Read the model definition and answer for the solid it produces. Units are mm, in the model's axes. Face numbers are marked on the shaded views. A direction names the side the tool comes from. Give positions to 0.01 mm unless a question says otherwise; leave off trailing zeros. Order: outer loops, then holes, each group sorted by start corner. A loop starts at its lowest first (then second) coordinate and runs counter-clockwise, first axis right, second up. Notation, with made-up numbers: (26, -2.75) - (35, -2.75) arc R12 ccw to (35, 9.25) - close; hole circle Ø9 at (83, -22.75). An arc over 180 degrees is marked (long way). Write each question's results on one line, items separated by ' | '. Start each with the question number.
Q1. Find section A-A on z = -10.5. Give the vertices of the cut face in (x, y), and give its area (3 significant figures).
Q2. Find section B-B on y = 61. Give the vertices of the cut face in (x, z).
Q3. Find section C-C on x = 5. Give the vertices of the cut face in (y, z).
Q4. Find the intervals of material crossed by line 1 along Z through (x, y) = (4.5, 40); line 2 along Y through (x, z) = (-10, 13.5); line 3 along Y through (x, z) = (18, 23), in increasing order. Write a range as from..to.
Q5. For a pull along Z with two mould halves and no side action, classify the marked faces 4, 5, 6 and 7 as +Z half, -Z half, draft (parallel to the pull), parting line (faces both ways), or undercut.
Q6. Flat-ended cylindrical pins translate along their axes: P1, Ø1, axis at x = -0.5, z = 36.5, coming from the -Y side; P2, Ø10, axis at x = -8, z = 63, coming from the +Y side; P3, Ø1, axis at x = -18, y = 23.5, coming from the -Z side. Find the tip coordinate at first contact, or state that the pin passes through.
Q7. Find section D-D on y = 40. Give the vertices of the cut face in (x, z), and give its area (3 significant figures).
Q8. A tool of negligible diameter and unlimited length cuts with its end or side. For the marked faces 1, 2 and 3, from which of +Z, -Z, +X, -X, +Y, -Y can it reach the whole face along a straight path? Write none if from no direction.
from build123d import *

# Parameters (mm, degrees)
SKETCH1_W           = 50
SKETCH1_H           = 50
BOSS_EXTRUDE1_DEPTH = 100
SKETCH2_W           = 50
SKETCH2_H           = 50
BOSS_EXTRUDE2_DEPTH = 50
CUT_EXTRUDE1_DEPTH  = 50
CUT_EXTRUDE3_DEPTH  = 25
CUT_EXTRUDE4_DEPTH  = 25
CUT_EXTRUDE5_REACH  = 52
SKETCH6_W           = 30
SKETCH6_H           = 30


with BuildPart() as part:
    # Sketch1 → Boss-Extrude1 (new body)
    with BuildSketch(Plane(origin=(0, 0, 0), x_dir=(1, 0, 0), z_dir=(0, 1, 0))):
        Rectangle(SKETCH1_W, SKETCH1_H)
    extrude(amount=BOSS_EXTRUDE1_DEPTH)

    # Sketch2 → Boss-Extrude2 (add)
    with BuildSketch(Plane.XY.offset(25)):
        with Locations((0, 50)):
            Rectangle(SKETCH2_W, SKETCH2_H)
    extrude(amount=BOSS_EXTRUDE2_DEPTH)

    # Sketch3 → Cut-Extrude1 (cut)
    with BuildSketch(Plane.XY.offset(75)):
        with BuildLine():
            Line((8.4e-08, 75), (-25, 75))
            Line((-25, 75), (-25, 49.999999966))
            ThreePointArc((-25, 49.999999966), (-17.677669512, 67.677669547), (8.4e-08, 75))
        make_face()
        with BuildLine():
            Line((25, 75), (8.4e-08, 75))
            ThreePointArc((8.4e-08, 75), (17.677669559, 67.6776695), (25, 50))
            Line((25, 50), (25, 75))
        make_face()
        with BuildLine():
            Line((25, 25), (25, 50))
            ThreePointArc((25, 50), (17.677669509, 32.32233045), (-5.8e-08, 25))
            Line((-5.8e-08, 25), (25, 25))
        make_face()
        with BuildLine():
            ThreePointArc((-5.8e-08, 25), (-17.677669538, 32.322330479), (-25, 49.999999966))
            Line((-25, 49.999999966), (-25, 25))
            Line((-25, 25), (-5.8e-08, 25))
        make_face()
    extrude(amount=-CUT_EXTRUDE1_DEPTH, mode=Mode.SUBTRACT)

    # Sketch4 → Cut-Extrude3 (cut)
    with BuildSketch(Plane(origin=(0, 100, 0), x_dir=(1, 0, 0), z_dir=(0, 1, 0))):
        with BuildLine():
            ThreePointArc((0, -25), (-17.67766954, -17.677669519), (-25, 3e-08))
            Line((-25, 3e-08), (-25, -25))
            Line((-25, -25), (0, -25))
        make_face()
        with BuildLine():
            Line((0, 25), (-25, 25))
            Line((-25, 25), (-25, 3e-08))
            ThreePointArc((-25, 3e-08), (-17.677669519, 17.67766954), (0, 25))
        make_face()
        with BuildLine():
            Line((25, 25), (0, 25))
            ThreePointArc((0, 25), (17.67766953, 17.67766953), (25, 0))
            Line((25, 0), (25, 25))
        make_face()
        with BuildLine():
            Line((25, -25), (25, 0))
            ThreePointArc((25, 0), (17.67766953, -17.67766953), (0, -25))
            Line((0, -25), (25, -25))
        make_face()
    extrude(amount=-CUT_EXTRUDE3_DEPTH, mode=Mode.SUBTRACT)

    # Sketch5 → Cut-Extrude4 (cut)
    with BuildSketch(Plane.XZ):
        with BuildLine():
            Line((-2e-08, 25), (-25, 25))
            Line((-25, 25), (-25, 1e-09))
            ThreePointArc((-25, 1e-09), (-17.677669536, 17.677669523), (-2e-08, 25))
        make_face()
        with BuildLine():
            Line((25, 25), (-2e-08, 25))
            ThreePointArc((-2e-08, 25), (17.677669523, 17.677669537), (25, 0))
            Line((25, 0), (25, 25))
        make_face()
        with BuildLine():
            Line((25, -25), (25, 0))
            ThreePointArc((25, 0), (17.67766952, -17.677669539), (-2.6e-08, -25))
            Line((-2.6e-08, -25), (25, -25))
        make_face()
        with BuildLine():
            ThreePointArc((-2.6e-08, -25), (-17.677669539, -17.67766952), (-25, 1e-09))
            Line((-25, 1e-09), (-25, -25))
            Line((-25, -25), (-2.6e-08, -25))
        make_face()
    extrude(amount=-CUT_EXTRUDE4_DEPTH, mode=Mode.SUBTRACT)

    # Sketch6 → Cut-Extrude5 (cut, up to next)
    with BuildSketch(Plane.ZY.offset(25), mode=Mode.PRIVATE) as cut_extrude5_sk1:
        with Locations((0, 50)):
            Rectangle(SKETCH6_W, SKETCH6_H)
    cut_extrude5_tool1 = extrude(cut_extrude5_sk1.sketch, amount=-CUT_EXTRUDE5_REACH, mode=Mode.PRIVATE) & part.part
    add(cut_extrude5_tool1.solids().sort_by_distance((-25, 50, 0))[0], mode=Mode.SUBTRACT)


solid = part.part
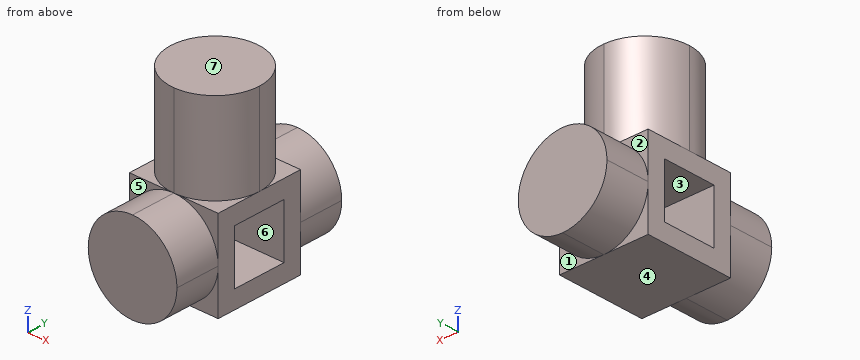
Working result:
1) outline: (-25, 25) - (-22.69, 25) - (-22.69, 0) - (22.69, 0) - (22.69, 25) - (25, 25) - (25, 35) - (-25, 35) - close; (-25, 65) - (25, 65) - (25, 75) - (22.69, 75) - (22.69, 100) - (-22.69, 100) - (-22.69, 75) - (-25, 75) - close | area: 3,270 mm²
2) outline: (-25, -25) - (25, -25) - (25, -15) - (-25, -15) - close; (-25, 15) - (25, 15) - (25, 25) - (22.45, 25) - (22.45, 75) - (-22.45, 75) - (-22.45, 25) - (-25, 25) - close
3) outline: (0, -24.49) - (25, -24.49) - (25, -25) - (75, -25) - (75, -24.49) - (100, -24.49) - (100, 24.49) - (75, 24.49) - (75, 25) - (74.49, 25) - (74.49, 75) - (25.51, 75) - (25.51, 25) - (25, 25) - (25, 24.49) - (0, 24.49) - close; hole (35, -15) - (65, -15) - (65, 15) - (35, 15) - close
4) line 1: -25..-15, 15..75 | line 2: 0..35, 65..100 | line 3: 25..75
5) face 4: -Z half | face 5: draft | face 6: undercut | face 7: +Z half
6) P1: y = 25 | P2: y = 74.82 | P3: z = -17.85
7) outline: (-25, -25) - (25, -25) - (25, -15) - (-25, -15) - close; (-25, 15) - (25, 15) - (25, 25) - (22.91, 25) - (22.91, 75) - (-22.91, 75) - (-22.91, 25) - (-25, 25) - close | area: 3,290 mm²
8) face 1: -Z, +X, +Y | face 2: +Z, -X, +Y | face 3: +X, -X
